Geometry check sheet. Reference: drawing and pictorial views, mm from the part's lowest x, y, z. A direction names the side the tool comes from. Coordinates: 2 decimals unless noted, no trailing zeros. Write each loop counter-clockwise with the first axis right and the second up, starting at its lowest first coordinate (ties: lowest second). Pieces come first, ordered by that corner, then holes. Notation, with made-up numbers: (31.25, 72.5) -> (36.25, 72.5) arc R30 ccw to (36.25, 97.5) -> close; hole circle Ø7 at (11.25, 74). An arc over 180 degrees is marked (long way). Answer in a Markdown table with one row per item.
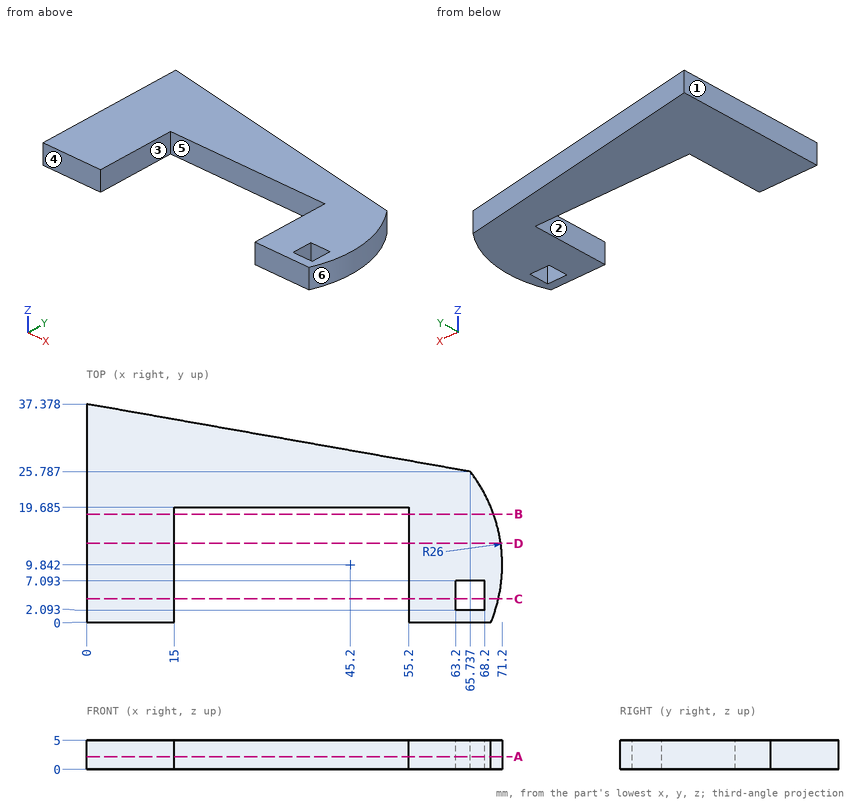
1. Depth check by flat-ended pin: P1, Ø3, axis at x = 46.5, z = 3, coming from the -Y side (1 decimal); P2, Ø2.5, axis at y = 14, z = 3, coming from the +X side. Enter the tip coordinate at first touch or a pass-through.
Geometry says:
| item | result |
|---|---|
| P1 | y = 19.7 |
| P2 | x = 71.04 |
2. Thickness scan on line 1 (X direction, y = 6, z = 0.5) (1 decimal); line 2 (X direction, y = 10.5, z = 2.3); line 3 (X direction, y = 18, z = 4.7). Record the ranges inside material, lowest first. Write a range as from..to.
Geometry says:
| item | result |
|---|---|
| line 1 | 0..15, 55.2..63.2, 68.2..70.9 |
| line 2 | 0..15, 55.2..71.19 |
| line 3 | 0..15, 55.2..69.89 |
3. Section check C-C, the plane y = 4. Record the boundary of the cut face in (x, z) (1 decimal).
Geometry says:
| item | result |
|---|---|
| outline | (0, 0) -> (15, 0) -> (15, 5) -> (0, 5) -> close; (55.2, 0) -> (63.2, 0) -> (63.2, 5) -> (55.2, 5) -> close; (68.2, 0) -> (70.5, 0) -> (70.5, 5) -> (68.2, 5) -> close |
4. Section check B-B, the plane y = 18.5. Record the boundary of the cut face in (x, z).
Geometry says:
| item | result |
|---|---|
| outline | (0, 0) -> (15, 0) -> (15, 5) -> (0, 5) -> close; (55.2, 0) -> (69.72, 0) -> (69.72, 5) -> (55.2, 5) -> close |
5. Section check D-D, the plane y = 13.5. Record the boundary of the cut face in (x, z).
Geometry says:
| item | result |
|---|---|
| outline | (0, 0) -> (15, 0) -> (15, 5) -> (0, 5) -> close; (55.2, 0) -> (70.94, 0) -> (70.94, 5) -> (55.2, 5) -> close |
6. Mould release check, pull along X, two halves, no side actions. Record for the marked faces 3, 4, 5 and 6: released by +X, released by -X, zero draft, split by the parting line, or undercut.
Geometry says:
| item | result |
|---|---|
| face 3 | undercut |
| face 4 | zero draft |
| face 5 | undercut |
| face 6 | released by +X |
7. Tool access check on the marked faces 1 and 2. Record the directions out of +Z, -Z, +X, -X, +Y, -Y that give a thin tool (end or side, any length) a straight path to the whole face; none if there is none.
Geometry says:
| item | result |
|---|---|
| face 1 | +Z, -Z, -X, +Y, -Y |
| face 2 | +Z, -Z, -Y |
8. Section check A-A, the plane z = 2.2. Record the boundary of the cut face in (x, y) (1 decimal), plus the area to 3 significant figures.
Geometry says:
| item | result |
|---|---|
| outline | (0, 0) -> (15, 0) -> (15, 19.7) -> (55.2, 19.7) -> (55.2, 0) -> (69.3, 0) arc R26 ccw to (65.7, 25.8) -> (0, 37.4) -> close; hole (63.2, 2.1) -> (68.2, 2.1) -> (68.2, 7.1) -> (63.2, 7.1) -> close |
| area | 1,370 mm^2 |
